Verification items for the finished model (mm, model axes). Face numbers are marked on the shaded views. Coordinates: 2 decimals unless noted, no trailing zeros. Order: outer loops, then holes, each group sorted by start corner. A loop starts at its lowest first (then second) coordinate and runs counter-clockwise, first axis right, second up.
Q1. Draft check along Y on the marked faces 1, 2, 3 and 4. Enter one of: pulls with the +Y half, pulls with the -Y half, needs draft (parallel to the pull), parting line crosses it, or undercut.
Q2. Depth check by flat-ended pin: P1, Ø1.3, axis at x = -44.5, y = 15.5, coming from the -Z side; P2, Ø2, axis at x = -45.5, z = 3, coming from the -Y side; P3, Ø8, axis at x = -19, y = -6, coming from the -Z side; P4, Ø1, axis at y = 22, z = -6.5, coming from the -X side. Enter the tip coordinate at first touch or a pass-through.
Q3. Cross-section at B-B, the plane x = 24. Record the boundary of the cut face in (y, z).
Q4. Thickness scan on line 1 (Y direction, x = 14, z = -6.25); line 2 (X direction, y = -3, z = 3.5); line 3 (Z direction, x = -44, y = -13). Record the ranges inside material, lowest first.
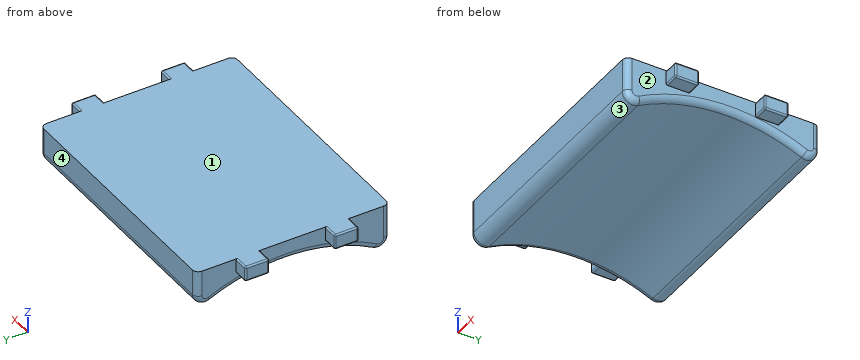
from build123d import *

# Parameters (mm, degrees)
CROQUIS1_W              = 85
CROQUIS1_H              = 65
SALIENTE_EXTRUIR1_DEPTH = 5
CROQUIS3_W              = 5
CROQUIS3_H              = 8
SALIENTE_EXTRUIR3_DEPTH = 5
SALIENTE_EXTRUIR2_DEPTH = 85
REDONDEO1_R             = 3.5
REDONDEO2_R             = 2
REDONDEO3_R             = 0.5


with BuildPart() as part:
    # Croquis1 → Saliente-Extruir1 (new body)
    with BuildSketch(Plane.XY):
        Rectangle(CROQUIS1_W, CROQUIS1_H)
    extrude(amount=SALIENTE_EXTRUIR1_DEPTH)

    # Croquis3 → Saliente-Extruir3 (add)
    with BuildSketch(Plane(origin=(42.5, 0, 0), x_dir=(0, 0, -1), z_dir=(1, 0, 0))):
        with Locations((-2.5, 15)):
            Rectangle(CROQUIS3_W, CROQUIS3_H)
        with Locations((-2.5, -15)):
            Rectangle(CROQUIS3_W, CROQUIS3_H)
    saliente_extruir3 = extrude(amount=SALIENTE_EXTRUIR3_DEPTH)

    # Simetría1: Saliente-Extruir3 across plane
    add(saliente_extruir3.mirror(Plane(origin=(0, 0, 0), x_dir=(0, 0, 1), z_dir=(1, 0, 0))))

    # Croquis2 → Saliente-Extruir2 (add)
    with BuildSketch(Plane(origin=(42.5, 0, 0), x_dir=(0, 0, -1), z_dir=(1, 0, 0))):
        with BuildLine():
            Line((0, 32.5), (9.313409495, 32.5))
            ThreePointArc((9.313409495, 32.5), (1.570605068, -0.446088635), (12.430740563, -32.5))
            Line((12.430740563, -32.5), (0, -32.5))
            Line((0, -32.5), (0, 32.5))
        make_face()
    extrude(amount=-SALIENTE_EXTRUIR2_DEPTH)

    # Redondeo1
    redondeo1_edges = [part.edges().sort_by_distance(p)[0] for p in [
        (0, 32.5, -9.313409495),
        (0, -32.5, -12.430740563),
    ]]
    fillet(redondeo1_edges, radius=REDONDEO1_R)

    # Redondeo2
    redondeo2_edges = [part.edges().sort_by_distance(p)[0] for p in [
        (-42.5, 32.5, 0.676379496),
        (42.5, 32.5, 0.676379496),
        (42.5, -32.5, -0.571361271),
        (-42.5, -32.5, -0.571361271),
        (42.5, -0.143625132, -1.556845408),
        (42.5, 30.904700663, -6.583584888),
        (42.5, -30.776719103, -9.158227347),
        (-42.5, -0.143625132, -1.556845408),
        (-42.5, 30.904700663, -6.583584888),
        (-42.5, -30.776719103, -9.158227347),
    ]]
    fillet(redondeo2_edges, radius=REDONDEO2_R)

    # Redondeo3
    redondeo3_edges = [part.edges().sort_by_distance(p)[0] for p in [
        (45, 19, 5),
        (45, 11, 5),
        (45, 11, 0),
        (45, 19, 0),
        (47.5, 15, 5),
        (47.5, 11, 2.5),
        (47.5, 15, 0),
        (47.5, 19, 2.5),
        (45, -19, 5),
        (45, -19, 0),
        (45, -11, 0),
        (45, -11, 5),
        (47.5, -19, 2.5),
        (47.5, -15, 0),
        (47.5, -11, 2.5),
        (47.5, -15, 5),
        (-47.5, 15, 5),
        (-45, 11, 5),
        (-47.5, 19, 2.5),
        (-45, 19, 5),
        (-47.5, 15, 0),
        (-45, 19, 0),
        (-47.5, 11, 2.5),
        (-45, 11, 0),
        (-47.5, -19, 2.5),
        (-45, -19, 0),
        (-47.5, -15, 5),
        (-45, -19, 5),
        (-47.5, -11, 2.5),
        (-45, -11, 5),
        (-47.5, -15, 0),
        (-45, -11, 0),
    ]]
    fillet(redondeo3_edges, radius=REDONDEO3_R)


solid = part.part
Check values:
1. face 1: needs draft
1. face 2: undercut
1. face 3: parting line crosses it
1. face 4: pulls with the +Y half
2. P1: stops at z = 0
2. P2: stops at y = -19
2. P3: stops at z = -2.78
2. P4: passes through
3. outline: (-32.5, -6.14) arc R3.5 ccw to (-27.3, -9.2) arc R61.5 cw to (27.57, -6.84) arc R3.5 ccw to (32.5, -3.65) - (32.5, 5) - (-32.5, 5) - close
4. line 1: y = -32.5 to -21.2, 26.2 to 31.34
4. line 2: x = -42.5 to 42.5
4. line 3: z = 0 to 5
